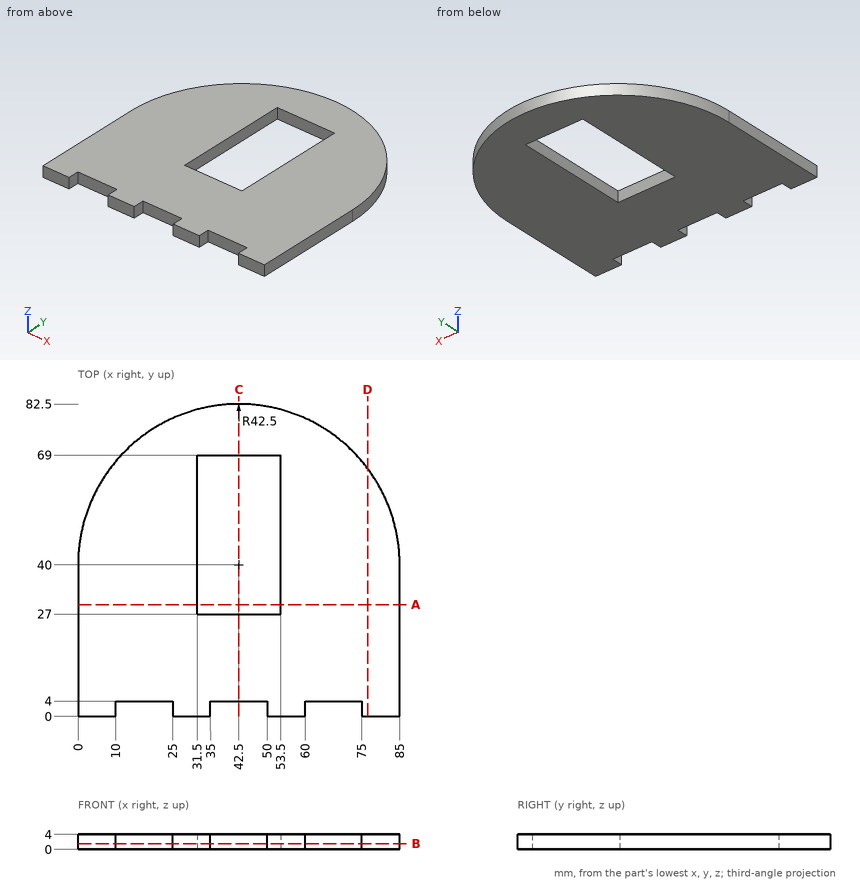
Answer from the drawing. Dimensions are ordinates in mm from the lowest x, y and z of the part. Give positions to 0.01 mm unless a question says otherwise; leave off trailing zeros. Write each loop counter-clockwise with the first axis right and the second up, starting at its lowest first coordinate (ties: lowest second). Pieces come first, ordered by that corner, then holes.
1) Find the intervals of material crossed by L1, parallel to X at y = 31, z = 3.8; L2, parallel to X at y = 47, z = 1.95; L3, parallel to Y at x = 36, z = 3.65, in increasing order.
2) Section A-A (y = 29.5) is taken. Write down the section's boundary in (x, z).
3) Given P1, Ø2, axis at x = 39.5, z = 2.5, coming from the +Y side; P2, Ø1.2, axis at x = 20.5, z = 1.5, coming from the -Y side; P3, Ø2, axis at y = 53, z = 1.5, coming from the +X side, each flat-ended and moving along its own axis, determine where each tip first touches the part or whether it passes through.
4) Section C-C (x = 42.5) is taken. Write down the section's boundary in (y, z).
5) Section D-D (x = 76.5) is taken. Write down the section's boundary in (y, z), and give its area (3 significant figures).
6) Section B-B (z = 1.5) is taken. Write down the section's boundary in (x, y), and give its area (3 significant figures).
Response:
1. L1: x = 0 to 31.5, 53.5 to 85
1. L2: x = 0.58 to 31.5, 53.5 to 84.42
1. L3: y = 4 to 27, 69 to 82
2. outline: (0, 0) - (31.5, 0) - (31.5, 4) - (0, 4) - close; (53.5, 0) - (85, 0) - (85, 4) - (53.5, 4) - close
3. P1: stops at y = 82.45
3. P2: stops at y = 4
3. P3: stops at x = 83.27
4. outline: (4, 0) - (27, 0) - (27, 4) - (4, 4) - close; (69, 0) - (82.5, 0) - (82.5, 4) - (69, 4) - close
5. outline: (0, 0) - (65.5, 0) - (65.5, 4) - (0, 4) - close
5. area: 262 mm2
6. outline: (0, 0) - (10, 0) - (10, 4) - (25, 4) - (25, 0) - (35, 0) - (35, 4) - (50, 4) - (50, 0) - (60, 0) - (60, 4) - (75, 4) - (75, 0) - (85, 0) - (85, 40) arc R42.5 ccw to (0, 40) - close; hole (31.5, 27) - (53.5, 27) - (53.5, 69) - (31.5, 69) - close
6. area: 5,130 mm2
